Check sheet for the modelled part. Datum: model origin and axes. Units: mm. Round coordinates to 2 decimals unless told otherwise and drop trailing zeros. Order: outer loops, then holes, each group sorted by start corner. A loop starts at its lowest first (then second) coordinate and runs counter-clockwise, first axis right, second up.
Q1. Cross-section at D-D on x = -29.5. Record the cut outline in (y, z), then the cut area to 3 significant figures.
Q2. Cross-section at C-C on z = 163.7. Record the cut outline in (x, y).
Q3. Scan lines: probe 1 along Y at (x, z) = (2.5, 164); probe 2 along Y at (x, z) = (-7.5, 164.5); probe 3 along X at (y, z) = (102.5, 162.8). Record each from-to range of solid material in increasing order.
Q4. Cross-section at A-A on x = 2.5. Record the cut outline in (y, z), then the cut area to 3 significant figures.
Q5. Cross-section at B-B on y = 84. Record the cut outline in (x, z), then the cut area to 3 significant figures.
Q6. Depth check by flat-ended pin: P1, Ø1, axis at y = 92, z = 164.5, coming from the -X side. Enter the tip coordinate at first touch or a pass-through.
Q7. Mould release check, pull along X, two halves, no side actions. Record for faces 1 (the flat face through (49.552, 102.18, 163.479)), 2 (the flat face through (1, 70, 163)), 3 (the cylindrical face through (3.75, 147.35, 163.48)), 4 (the cylindrical face through (17.418, 129.018, 163.479)): +X half, -X half, draft (parallel to the pull), parting line (faces both ways), or undercut.
from build123d import *

# Parameters (mm, degrees)
SKETCH1_R           = 27.75
BOSS_EXTRUDE1_DEPTH = 3


with BuildPart() as part:
    # Sketch1 → Boss-Extrude1 (new body)
    with BuildSketch(Plane.XY.offset(162)):
        with BuildLine():
            Line((-45.305021967, 70), (-20, 70))
            Line((-20, 70), (20, 70))
            Line((20, 70), (45.305021967, 70))
            Line((45.305021967, 70), (49.846930848, 70))
            ThreePointArc((49.846930848, 70), (57.376653748, 74.070165008), (58.0958845, 82.599272656))
            Line((58.0958845, 82.599272656), (40.765979439, 122.316625933))
            ThreePointArc((40.765979439, 122.316625933), (3.077668906, 147.366003385), (-35.28933022, 123.36905692))
            Line((-35.28933022, 123.36905692), (-54.331701831, 82.826144007))
            ThreePointArc((-54.331701831, 82.826144007), (-53.782712085, 74.174821043), (-46.185498909, 70))
            Line((-46.185498909, 70), (-45.305021967, 70))
        make_face()
        with Locations((2.5, 105.61875)):
            Circle(SKETCH1_R, mode=Mode.SUBTRACT)
    extrude(amount=BOSS_EXTRUDE1_DEPTH)


solid = part.part
Results found:
1. outline: (70, 162) - (132.44, 162) - (132.44, 165) - (70, 165) - close
1. area: 187 mm2
2. outline: (-54.33, 82.83) arc R9 ccw to (-46.19, 70) - (49.85, 70) arc R9 ccw to (58.1, 82.6) - (40.77, 122.32) arc R41.75 ccw to (-35.29, 123.37) - close; hole circle Ø55.5 at (2.5, 105.62)
3. probe 1: y = 70 to 77.87, 133.37 to 147.37
3. probe 2: y = 70 to 79.73, 131.5 to 146.15
3. probe 3: x = -45.09 to -25.07, 30.07 to 49.41
4. outline: (70, 162) - (77.87, 162) - (77.87, 165) - (70, 165) - close; (133.37, 162) - (147.37, 162) - (147.37, 165) - (133.37, 165) - close
4. area: 65.6 mm2
5. outline: (-53.78, 162) - (-14.9, 162) - (-14.9, 165) - (-53.78, 165) - close; (19.9, 162) - (57.48, 162) - (57.48, 165) - (19.9, 165) - close
5. area: 229 mm2
6. P1: stops at x = -50.26
7. face 1: +X half
7. face 2: draft
7. face 3: parting line
7. face 4: undercut
